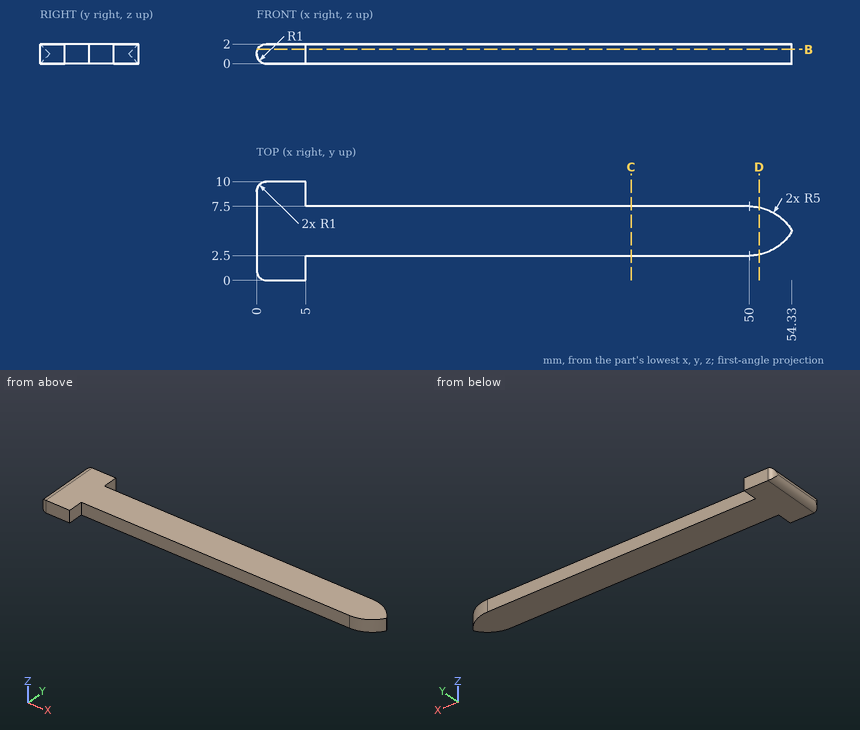
Source: three-view drawing plus pictorial views. Frame: mm from the lowest corner of the part. Round coordinates to 2 decimals unless told otherwise and drop trailing zeros. Loops run counter-clockwise (first coordinate to the right, second up) from the corner with the lowest first, then second, coordinate; pieces in that order, holes last.
Q1. Pin query (flat end, axial travel): P1, Ø1, axis at x = 24, z = 0.5, coming from the +Y side. Return the tip coordinate at first contact, or that it passes through.
Q2. Section B-B on z = 1.45. Return loops of the section in (x, y).
Q3. Section D-D on x = 51. Return loops of the section in (y, z).
Q4. Material intervals for L1, parallel to Y at x = 36, z = 1.15; L2, parallel to X at y = 6.75, z = 0.5 (1 decimal); L3, parallel to X at y = 5, z = 0.4, sorted ascending.
Q5. Section C-C on x = 38. Return loops of the section in (y, z).
Evaluation:
1. P1: stops at y = 7.5
2. outline: (0.11, 0.55) arc R1 ccw to (1, 0) - (5, 0) - (5, 2.5) - (50, 2.5) arc R5 ccw to (54.33, 5) arc R5 ccw to (50, 7.5) - (5, 7.5) - (5, 10) - (1, 10) arc R1 ccw to (0.11, 9.45) - close
3. outline: (2.6, 0) - (7.4, 0) - (7.4, 2) - (2.6, 2) - close
4. L1: y = 2.5 to 7.5
4. L2: x = 0.1 to 52.6
4. L3: x = 0.2 to 54.33
5. outline: (2.5, 0) - (7.5, 0) - (7.5, 2) - (2.5, 2) - close
